Geometry check sheet. Reference: drawing and pictorial views, mm from the part's lowest x, y, z. Give positions to 0.01 mm unless a question says otherwise; leave off trailing zeros. Order: outer loops, then holes, each group sorted by start corner. A loop starts at its lowest first (then second) coordinate and runs counter-clockwise, first axis right, second up.
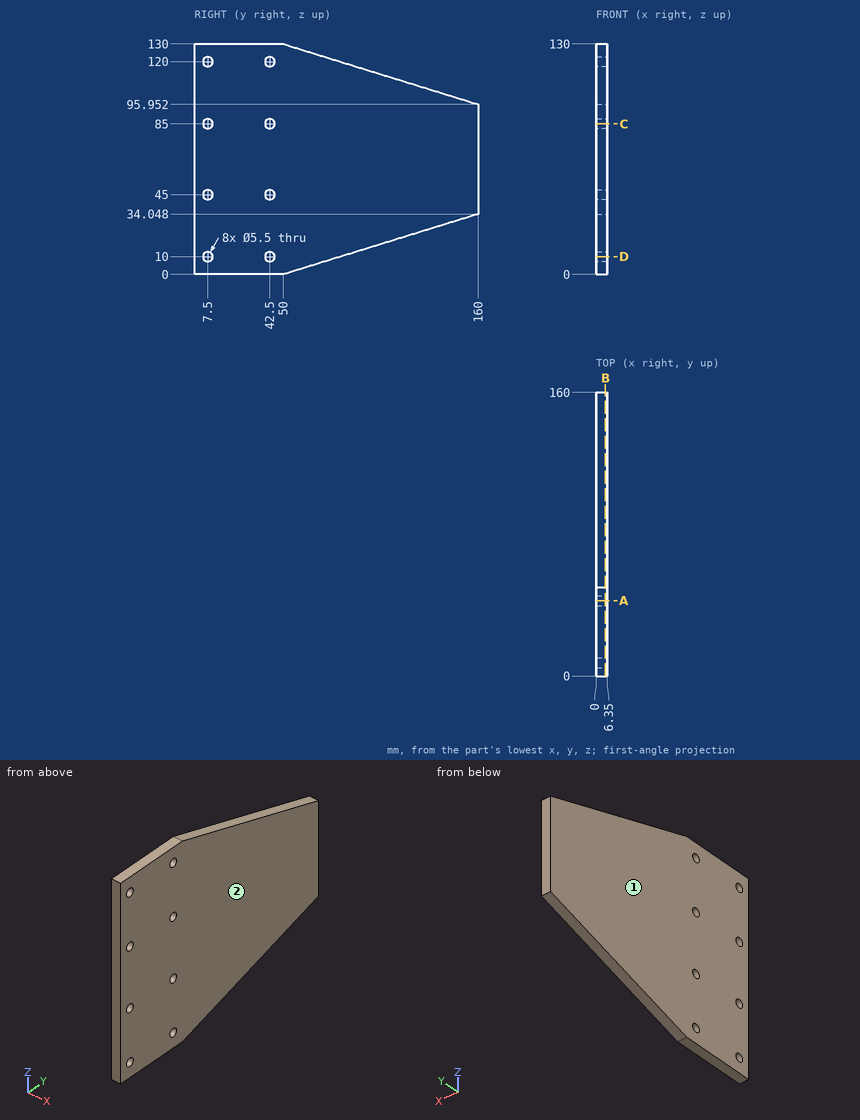
1) Material ranges on L1, parallel to Y at x = 1.75, z = 85; L2, parallel to Z at x = 5, y = 126.5; L3, parallel to Z at x = 1.5, y = 99.5, recorded low to high.
Recorded:
L1: y = 0 to 4.75, 10.25 to 39.75, 45.25 to 160
L2: z = 23.68 to 106.32
L3: z = 15.32 to 114.68
2) Section check B-B, the plane x = 5.25. State how many separate pieces and enclosed holes the cut face has, then the cut area to 3 significant figures.
Recorded:
separate pieces: 1
enclosed holes: 8
area: 16,900 mm2
3) Draft check along X on the marked faces 1 and 2. Enter one of: +X half, -X half, draft (parallel to the pull), parting line (faces both ways), or undercut.
Recorded:
face 1: -X half
face 2: +X half
4) Section check C-C, the plane z = 85. Record the cut outline in (x, y), then the cut area to 3 significant figures.
Recorded:
outline: (0, 0) - (6.35, 0) - (6.35, 4.75) - (0, 4.75) - close; (0, 10.25) - (6.35, 10.25) - (6.35, 39.75) - (0, 39.75) - close; (0, 45.25) - (6.35, 45.25) - (6.35, 160) - (0, 160) - close
area: 946 mm2
5) Section check D-D, the plane z = 10. Record the cut outline in (x, y), then the cut area to 3 significant figures.
Recorded:
outline: (0, 0) - (6.35, 0) - (6.35, 4.75) - (0, 4.75) - close; (0, 10.25) - (6.35, 10.25) - (6.35, 39.75) - (0, 39.75) - close; (0, 45.25) - (6.35, 45.25) - (6.35, 82.31) - (0, 82.31) - close
area: 453 mm2
6) Section check A-A, the plane y = 42.5. Record the cut outline in (x, z), then the cut area to 3 significant figures.
Recorded:
outline: (0, 0) - (6.35, 0) - (6.35, 7.25) - (0, 7.25) - close; (0, 12.75) - (6.35, 12.75) - (6.35, 42.25) - (0, 42.25) - close; (0, 47.75) - (6.35, 47.75) - (6.35, 82.25) - (0, 82.25) - close; (0, 87.75) - (6.35, 87.75) - (6.35, 117.25) - (0, 117.25) - close; (0, 122.75) - (6.35, 122.75) - (6.35, 130) - (0, 130) - close
area: 686 mm2
